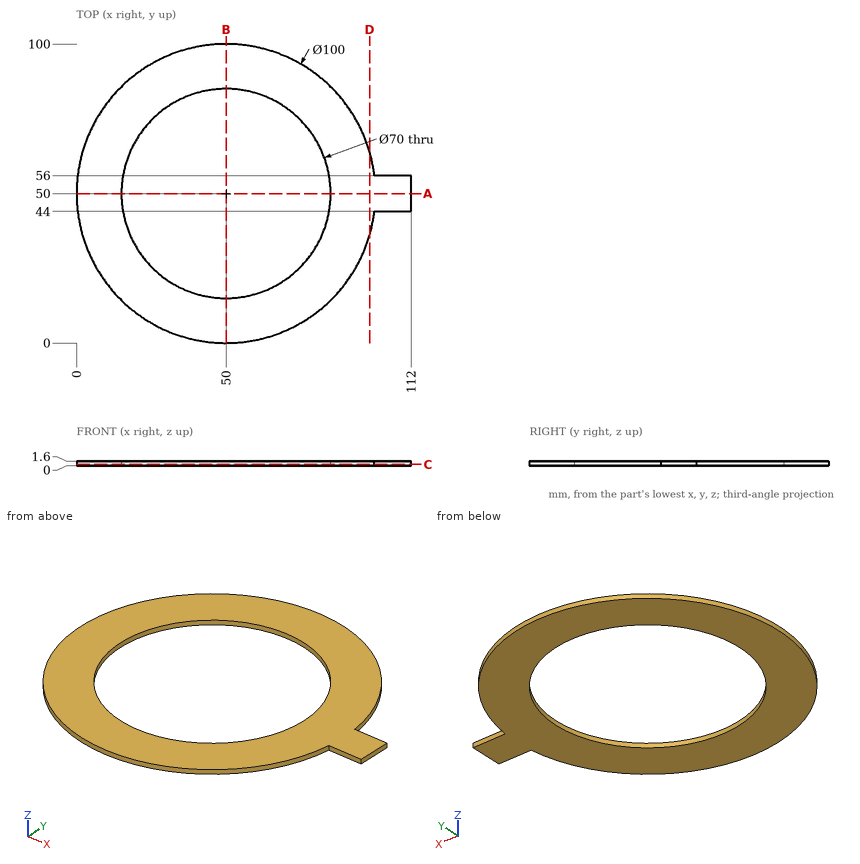
Part print with two shaded views. Sizes in mm from the minimum x, y, z corner. Coordinates: 2 decimals unless noted, no trailing zeros. Write each loop counter-clockwise with the first axis right and the second up, starting at its lowest first coordinate (ties: lowest second). Pieces come first, ordered by that corner, then holes.
(1) Drill centre lines: line 1 (Y direction, x = 50.5, z = 0.4); line 2 (Y direction, x = 104, z = 0.2); line 3 (X direction, y = 27, z = 1.1). Where is each one in solid material? Low to high.
(2) Cut at D-D on x = 98. List the corners of the cut face in (y, z), and give its area (3 significant figures).
(3) Cut at C-C on z = 0.5. List the corners of the cut face in (x, y), and give its area (3 significant figures).
(4) Cut at A-A on y = 50. List the corners of the cut face in (x, z).
(5) Pin check, flat tips, straight feed: pin 1 Ø0.5 at (x, z) = (105.5, 1) entering from +Y; pin 2 Ø6 at (x, y) = (12, 34) entering from -Z. Stop position of each tip, or through.
(6) Cut at B-B on x = 50. List the corners of the cut face in (y, z), and give its area (3 significant figures).
Working result:
1. line 1: y = 0 to 15, 85 to 100
1. line 2: y = 44 to 56
1. line 3: x = 5.6 to 23.62, 76.38 to 94.4
2. outline: (36, 0) - (64, 0) - (64, 1.6) - (36, 1.6) - close
2. area: 44.8 mm2
3. outline: (99.64, 44) - (112, 44) - (112, 56) - (99.64, 56) arc R50 ccw (long way) to start; hole circle Ø70 at (50, 50)
3. area: 4,150 mm2
4. outline: (0, 0) - (15, 0) - (15, 1.6) - (0, 1.6) - close; (85, 0) - (112, 0) - (112, 1.6) - (85, 1.6) - close
5. pin 1: stops at y = 56
5. pin 2: stops at z = 0
6. outline: (0, 0) - (15, 0) - (15, 1.6) - (0, 1.6) - close; (85, 0) - (100, 0) - (100, 1.6) - (85, 1.6) - close
6. area: 48.0 mm2
